```python
from build123d import *

# Parameters (mm, degrees)
SKETCH1_R                = 80
BOSS_EXTRUDE1_DEPTH      = 1.6
SKETCH2_R                = 2.3
CUT_EXTRUDE1_DEPTH       = 1.6
M2_CLEARANCE_HOLE2_D     = 2.2
M2_CLEARANCE_HOLE2_DEPTH = 6
M2_CLEARANCE_HOLE2_TIP   = 0.660946681
SKETCH9_R                = 30.8
BOSS_EXTRUDE2_DEPTH      = 18.86
SKETCH10_R               = 1.5
BOSS_EXTRUDE3_DEPTH      = 4
SKETCH11_R               = 0.7
BOSS_EXTRUDE4_DEPTH      = 3.8


with BuildPart() as part:
    # Sketch1 → Boss-Extrude1 (new body)
    with BuildSketch(Plane(origin=(0, 0, 0), x_dir=(1, 0, 0), z_dir=(0, 1, 0))):
        Circle(SKETCH1_R)
    extrude(amount=BOSS_EXTRUDE1_DEPTH)

    # Sketch2 → Cut-Extrude1 (cut)
    with BuildSketch(Plane(origin=(0, 1.6, 0), x_dir=(1, 0, 0), z_dir=(0, 1, 0))):
        Circle(SKETCH2_R)
    extrude(amount=-CUT_EXTRUDE1_DEPTH, mode=Mode.SUBTRACT)

    # M2 Clearance Hole2
    with Locations(Plane(origin=(0, 1.6, 0), x_dir=(1, 0, 0), z_dir=(0, 1, 0))):
        with Locations((0, 76), (76, 0), (-76, 0)):
            Hole(M2_CLEARANCE_HOLE2_D / 2, depth=M2_CLEARANCE_HOLE2_DEPTH)
            with Locations((0, 0, -(M2_CLEARANCE_HOLE2_DEPTH + M2_CLEARANCE_HOLE2_TIP / 2))):  # 118° drill point
                Cone(0, M2_CLEARANCE_HOLE2_D / 2, M2_CLEARANCE_HOLE2_TIP, mode=Mode.SUBTRACT)

    # Sketch9 → Boss-Extrude2 (add)
    with BuildSketch(Plane(origin=(0, 1.6, 0), x_dir=(1, 0, 0), z_dir=(0, 1, 0))):
        Circle(SKETCH9_R)
    extrude(amount=BOSS_EXTRUDE2_DEPTH)

    # Sketch10 → Boss-Extrude3 (add)
    with BuildSketch(Plane.XZ.offset(-1.6)):
        Circle(SKETCH10_R)
    extrude(amount=BOSS_EXTRUDE3_DEPTH)

    # Sketch11 → Boss-Extrude4 (add)
    with BuildSketch(Plane.XZ.offset(2.4)):
        Circle(SKETCH11_R)
    extrude(amount=BOSS_EXTRUDE4_DEPTH)


solid = part.part
```
Check sheet for the modelled part. Datum: model origin and axes. Units: mm. A direction names the side the tool comes from. Round coordinates to 2 decimals unless told otherwise and drop trailing zeros. Loops run counter-clockwise (first coordinate to the right, second up) from the corner with the lowest first, then second, coordinate; pieces in that order, holes last. Notation, with made-up numbers: (65, 71.25) -> (121, 71.25) arc R5 ccw to (121, 80.25) -> close; hole circle Ø7 at (-36.75, 2). An arc over 180 degrees is marked (long way). Answer in a Markdown table with one row per item.
Q1. Thickness scan on L1, parallel to Z at x = 0, y = 0.3; L2, parallel to Y at x = 54, z = 9; L3, parallel to Z at x = 2.5, y = 10.5. Record the ranges inside material, lowest first.
Data:
| item | result |
|---|---|
| L1 | z = -80 to -77.1, -74.9 to -2.3, -1.5 to 1.5, 2.3 to 80 |
| L2 | y = 0 to 1.6 |
| L3 | z = -30.7 to 30.7 |
Q2. Sectioned sample at A-A on z = 7. Enter the section's corners in (x, y), then the cut area to 3 significant figures.
Data:
| item | result |
|---|---|
| outline | (-79.69, 0) -> (79.69, 0) -> (79.69, 1.6) -> (29.99, 1.6) -> (29.99, 20.46) -> (-29.99, 20.46) -> (-29.99, 1.6) -> (-79.69, 1.6) -> close |
| area | 1,390 mm^2 |
Q3. Sectioned sample at D-D on z = -68.5. Enter the section's corners in (x, y).
Data:
| item | result |
|---|---|
| outline | (-41.32, 0) -> (41.32, 0) -> (41.32, 1.6) -> (-41.32, 1.6) -> close |
Q4. Release check for a two-part mould opening along X. For faces 1 (the face through (2, 1.6, 0)), 2 (the face through (-1, 1.6, 34)), 3 (the face through (-6.677, 10.898, 30.068)) record: released by +X, released by -X, zero draft, split by the parting line, or undercut.
Data:
| item | result |
|---|---|
| face 1 | undercut |
| face 2 | zero draft |
| face 3 | split by the parting line |
Q5. Sectioned sample at B-B on y = 15. Enter the section's corners in (x, z).
Data:
| item | result |
|---|---|
| outline | circle Ø61.6 at (0, 0) |
Q6. Set-up check for faces 4 (the face through (-1.825, 0.811, 1.4)), 5 (the face through (0, 20.46, 0)): record each of +Z, -Z, +X, -X, +Y, -Y from which the full face is reachable in a straight line by a thin tool's end or side.
Data:
| item | result |
|---|---|
| face 4 | -Y |
| face 5 | +Z, -Z, +X, -X, +Y |
Q7. Sectioned sample at C-C on x = -52. Enter the section's corners in (y, z).
Data:
| item | result |
|---|---|
| outline | (0, -60.79) -> (1.6, -60.79) -> (1.6, 60.79) -> (0, 60.79) -> close |
Q8. Go/stop test with flat-tipped pins: P1, Ø8, axis at x = 34, y = 3, coming from the -Z side; P2, Ø2, axis at x = -76, z = 0, coming from the -Y side; P3, Ø2.5, axis at x = 0, z = -76, coming from the +Y side. Record where each tip stops, or that it passes through.
Data:
| item | result |
|---|---|
| P1 | stops at z = -74.06 |
| P2 | passes through |
| P3 | stops at y = 1.6 |
